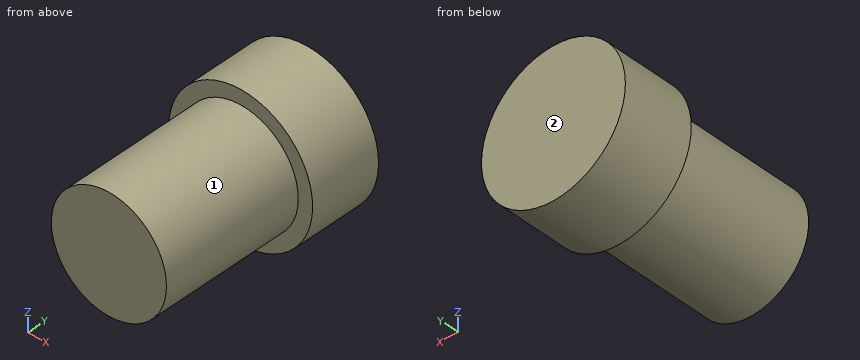
from build123d import *

# Parameters (mm, degrees)
F0_R          = 3.175
F1_DEPTH      = 6.35
F2_R          = 2.54
F3_DEPTH      = 6.35
F3_DEPTH_BACK = 12.7
F5_DEPTH      = 12.7
F6_W          = 10.36966
F6_H          = 6.35
F7_DEPTH      = 25.4


with BuildPart() as f1:
    # F0 (on Front) → F1 (new body)
    with BuildSketch(Plane.XZ):
        Circle(F0_R)
    extrude(amount=F1_DEPTH)

    # F2 (on face) → F3 (join, two sides)
    with BuildSketch(Plane.XZ.offset(6.35)) as f3_sk:
        Circle(F2_R)
    extrude(amount=F3_DEPTH)
    extrude(f3_sk.sketch, amount=-F3_DEPTH_BACK)

    # F4 (on Right) → F5 (cut)
    with BuildSketch(Plane.YZ):
        Polygon((8.097555, 3.648834), (-3.175, 3.868401), (-3.175, 0), (-3.175, -4.03599), (8.097555, -4.03599), align=None)
    extrude(amount=-F5_DEPTH, mode=Mode.SUBTRACT)

    # F6 (on face) → F7 (cut)
    with BuildSketch(Plane(origin=(0, 0, 0), x_dir=(0, -1, 0), z_dir=(-1, 0, 0))):
        with Locations((-2.00983, 0)):
            Rectangle(F6_W, F6_H)
    extrude(amount=-F7_DEPTH, mode=Mode.SUBTRACT)


solid = f1.part
Source: CAD feature listing. Evaluate the final solid. Frame: model axes, mm. Face numbers are marked on the shaded views. A direction names the side the tool comes from. Coordinates: 2 decimals unless noted, no trailing zeros. Loops run counter-clockwise (first coordinate to the right, second up) from the corner with the lowest first, then second, coordinate; pieces in that order, holes last. Notation, with made-up numbers: (58.25, -19.75) - (105.25, -19.75) arc R32 cw to (105.25, 19.25) - close; hole circle Ø9 at (26, 49). An arc over 180 degrees is marked (long way). Return JSON: item names as keys, results as strings.
Q1. Section C-C, the plane y = -5.25. Return loops of the section in (x, z) (3 decimals).
Results:
{"outline": "circle Ø6.35 at (0, 0)"}
Q2. Material intervals for line 1 along Y through (x, z) = (-2, -2.25) (3 decimals); line 2 along X through (y, z) = (-8, 2.25); line 3 along Z through (x, y) = (-1.5, -10), sorted ascending.
Results:
{"line 1": "-6.35 to -3.175", "line 2": "-1.18 to 1.18", "line 3": "-2.05 to 2.05"}
Q3. Contact query for flat-ended pins moving along their axis: P1, Ø1, axis at y = -11, z = 0, coming from the -X side; P2, Ø1.5, axis at y = -11.5, z = -1, coming from the +X side. Output: stop coordinate, or through.
Results:
{"P1": "x = -2.54", "P2": "x = 2.53"}
Q4. Section B-B, the plane z = 0. Return loops of the section in (x, y) (3 decimals).
Results:
{"outline": "(-3.175, -6.35) - (-2.54, -6.35) - (-2.54, -12.7) - (2.54, -12.7) - (2.54, -6.35) - (3.175, -6.35) - (3.175, -3.175) - (-3.175, -3.175) - close"}
Q5. Section D-D, the plane y = -11.25. Return loops of the section in (x, z), plus the area to 3 significant figures.
Results:
{"outline": "circle Ø5.08 at (0, 0)", "area": "20.3 mm2"}
Q6. Section A-A, the plane x = 0. Return loops of the section in (y, z) (3 decimals), plus the area to 3 significant figures.
Results:
{"outline": "(-12.7, -2.54) - (-6.35, -2.54) - (-6.35, -3.175) - (-3.175, -3.175) - (-3.175, 3.175) - (-6.35, 3.175) - (-6.35, 2.54) - (-12.7, 2.54) - close", "area": "52.4 mm2"}
Q7. Access query for the marked faces 1 and 2. Directions: +Z, -Z, +X, -X, +Y, -Y. A direction counts if a zero-diameter tool reaches every point of the face in a straight line with its end or side. Return the directions, or none.
Results:
{"face 1": "-Y", "face 2": "+Z, -Z, +X, -X, +Y"}
